Part print with two shaded views. Sizes in mm from the minimum x, y, z corner. A direction names the side the tool comes from. Round coordinates to 2 decimals unless told otherwise and drop trailing zeros. Order: outer loops, then holes, each group sorted by start corner. A loop starts at its lowest first (then second) coordinate and runs counter-clockwise, first axis right, second up. Notation, with made-up numbers: (70, 74) -> (126, 74) arc R24 cw to (126, 86) -> close; hole circle Ø1 at (-28.75, 55.5). An arc over 180 degrees is marked (long way). Use a Markdown table: item, result. Add a question column.
Item 1: Pin check, flat tips, straight feed: pin 1 (12 mm diameter, centred on x = 99.5, z = 20, fed in from -Y); pin 2 (25 mm diameter, centred on x = 56, y = 70, fed in from +Z); pin 3 (5 mm diameter, centred on x = 107, z = 38, fed in from +Y); pin 4 (1 mm diameter, centred on x = 74.5, y = 79, fed in from -Z). Stop position of each tip, or through.
Item 2: Slice it at A-A, the plane y = 36.5. Give the cut face in (x, z) (1 decimal), plus the area to 3 significant figures.
Item 3: Two-plate mould, pull along X, no slides. Class the marked faces 6, 7 and 8: released by +X, released by -X, zero draft, split by the parting line, or undercut.
Item 4: Slice it at D-D, the plane x = 24.5. Give the cut face in (y, z) (1 decimal).
Item 5: Probe L1, parallel to Y at x = 179, z = 37.5; L2, parallel to Z at x = 8, y = 64 (1 decimal); L3, parallel to X at y = 24, z = 7. List the from-to ranges inside material, lowest first.
Item 6: Slice it at B-B, the plane x = 45. Give the cut face in (y, z) (1 decimal), plus the area to 3 significant figures.
Item 7: 3-axis set-ups, long thin cutter, end or side, ignore diameter. For the marked faces 1, 2, 3, 4 and 5: which of +Z, -Z, +X, -X, +Y, -Y reach the whole face in a straight line?
Item 8: Slice it at C-C, the plane z = 22. Give the cut face in (x, y).
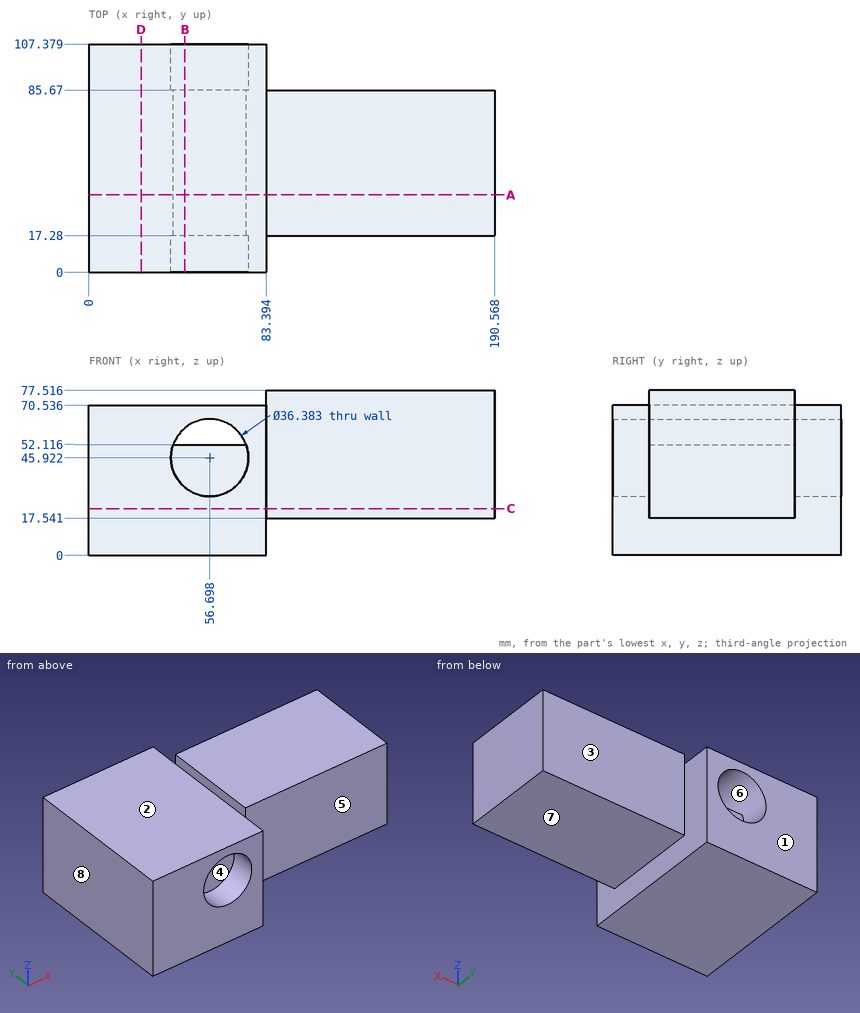
Check sheet entries:
| question | item | result |
|---|---|---|
| 1 | pin 1 | y = 17.28 |
| 1 | pin 2 | z = 70.54 |
| 1 | pin 3 | y = 85.67 |
| 1 | pin 4 | z = 0 |
| 2 | outline | (0, 0) -> (83.4, 0) -> (83.4, 17.5) -> (190.6, 17.5) -> (190.6, 77.5) -> (83.4, 77.5) -> (83.4, 70.5) -> (0, 70.5) -> close; hole (39.6, 52.1) -> (73.8, 52.1) arc R18.2 ccw to start |
| 2 | area | 12,000 mm2 |
| 3 | face 6 | undercut |
| 3 | face 7 | zero draft |
| 3 | face 8 | released by -X |
| 4 | outline | (0, 0) -> (107.4, 0) -> (107.4, 70.5) -> (0, 70.5) -> close |
| 5 | L1 | 17.28 to 85.67 |
| 5 | L2 | 0 to 70.5 |
| 5 | L3 | 0 to 83.39 |
| 6 | outline | (0, 0) -> (107.4, 0) -> (107.4, 32) -> (85.7, 32) -> (85.7, 52.1) -> (17.3, 52.1) -> (17.3, 32) -> (0, 32) -> close; (0, 59.9) -> (107.4, 59.9) -> (107.4, 70.5) -> (0, 70.5) -> close |
| 6 | area | 5,960 mm2 |
| 7 | face 1 | +Z, -Z, +X, -X, +Y |
| 7 | face 2 | +Z, -X, +Y, -Y |
| 7 | face 3 | +Z, -Z, +X, +Y |
| 7 | face 4 | -Y |
| 7 | face 5 | +Z, -Z, +X, -Y |
| 8 | outline | (0, 0) -> (83.39, 0) -> (83.39, 17.28) -> (190.57, 17.28) -> (190.57, 85.67) -> (83.39, 85.67) -> (83.39, 107.38) -> (0, 107.38) -> close |
